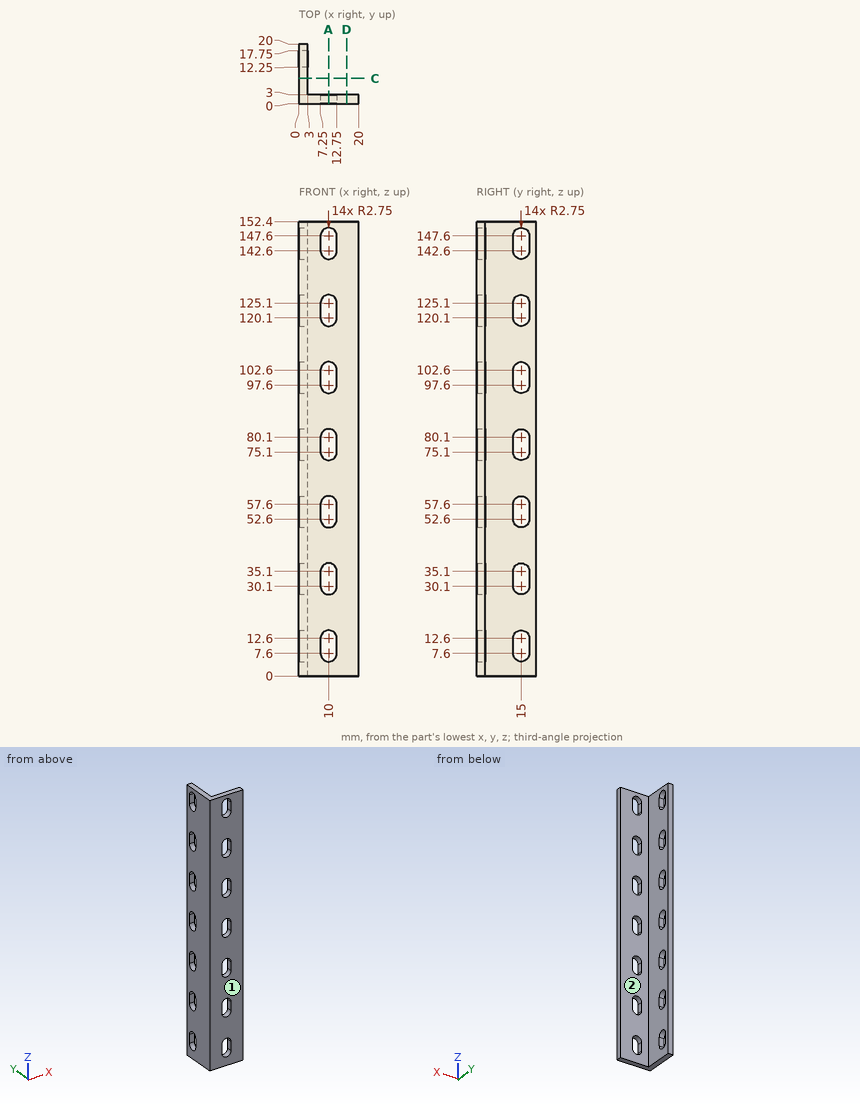
Can you work these out from the drawing? Everything is in mm from the part's minimum corner. A direction names the side the tool comes from. Coordinates: 2 decimals unless noted, no trailing zeros. Order: outer loops, then holes, each group sorted by start corner. A loop starts at its lowest first (then second) coordinate and runs counter-clockwise, first axis right, second up. Notation, with made-up numbers: (31, 65) -> (81, 65) arc R28 cw to (81, 93) -> close; hole circle Ø4 at (23, 75.5). An arc over 180 degrees is marked (long way). Return JSON: item names as keys, results as strings.
1) If we section it at A-A on x = 10: State how many separate pieces and enclosed holes the cut face has, plus the area to 3 significant figures.
Conclusion:
{"separate pieces": "8", "enclosed holes": "0", "area": "237 mm²"}
2) If we section it at C-C on y = 8.5: List the corners of the cut face in (x, z) for me.
Conclusion:
{"outline": "(0, 0) -> (3, 0) -> (3, 152.4) -> (0, 152.4) -> close"}
3) I'm going to push flat-ended pins straight in: P1, Ø1.5, axis at x = 16.5, z = 110.5, coming from the +Y side; P2, Ø0.9, axis at x = 1.5, z = 100.5, coming from the -Y side; P3, Ø10, axis at y = 9.5, z = 109.5, coming from the +X side. Where does each tip first touch, or does it pass through?
Conclusion:
{"P1": "stops at y = 3", "P2": "stops at y = 0", "P3": "stops at x = 3"}
4) On a 3-axis mill with a long thin cutter (end or side, diameter ignored), from which of +Z, -Z, +X, -X, +Y, -Y can I reach the whole of each face in a straight line? I mean the marked faces 1 and 2. Say none if no direction works.
Conclusion:
{"face 1": "+Z, -Z, +X, -X, -Y", "face 2": "+Z, -Z, +X, +Y"}
5) If I drill on probe 1 along X at (y, z) = (1.25, 143.5); probe 2 along Y at (x, z) = (1, 54); probe 3 along X at (y, z) = (11.75, 48.5), over which ranges is the centre line in solid material (lowest first)?
Conclusion:
{"probe 1": "x = 0 to 7.25, 12.75 to 20", "probe 2": "y = 0 to 12.25, 17.75 to 20", "probe 3": "x = 0 to 3"}
